The drawing under review shows one solid part. Ordinate dimensions are in mm from its lowest x, y, z. Coordinates: 2 decimals unless noted, no trailing zeros. Write each loop counter-clockwise with the first axis right and the second up, starting at its lowest first coordinate (ties: lowest second). Pieces come first, ordered by that corner, then holes.
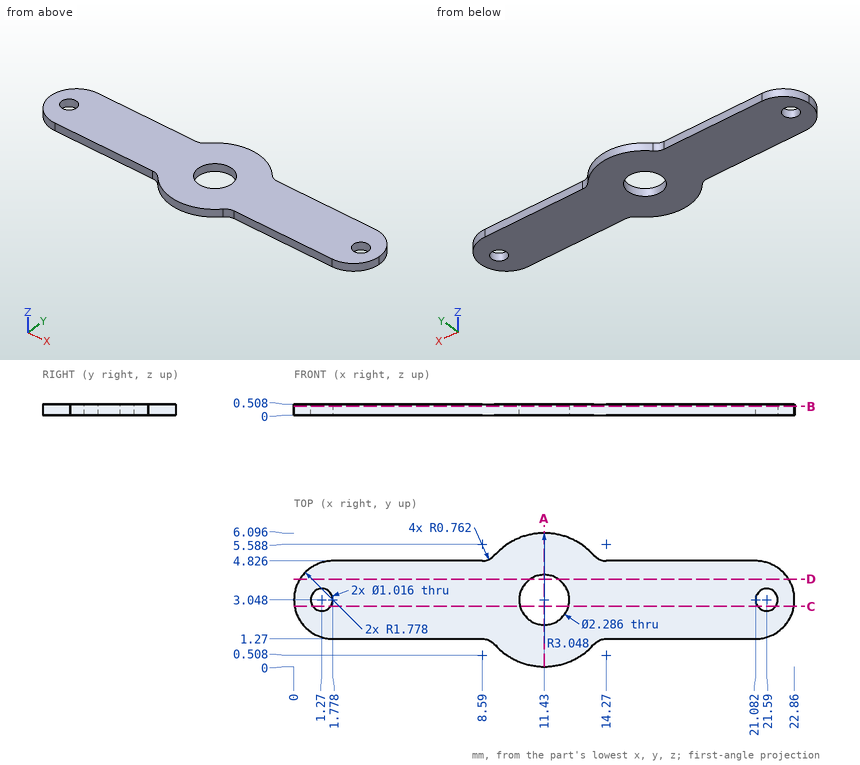
Q1. Add section C-C (y = 2.75). State the section outline as (x, z) points (1 decimal).
Ans:
outline: (0, 0) - (0.9, 0) - (0.9, 0.5) - (0, 0.5) - close; (1.7, 0) - (10.3, 0) - (10.3, 0.5) - (1.7, 0.5) - close; (12.5, 0) - (21.2, 0) - (21.2, 0.5) - (12.5, 0.5) - close; (22, 0) - (22.8, 0) - (22.8, 0.5) - (22, 0.5) - close
Q2. Add section D-D (y = 4). State the section outline as (x, z) points.
Ans:
outline: (0.28, 0) - (10.8, 0) - (10.8, 0.51) - (0.28, 0.51) - close; (12.06, 0) - (22.58, 0) - (22.58, 0.51) - (12.06, 0.51) - close
Q3. For probe 1 along Y at (x, z) = (11.43, 0.45) (3 decimals); probe 2 along Y at (x, z) = (21, 0.45); probe 3 along X at (y, z) = (3.5, 0.1), list the stretches that pass through material, from the lowest coordinate up.
Ans:
probe 1: y = 0 to 1.905, 4.191 to 6.096
probe 2: y = 1.27 to 4.83
probe 3: x = 0.06 to 1.04, 1.5 to 10.38, 12.48 to 21.36, 21.82 to 22.8
Q4. Add section B-B (z = 0.4). State the section outline as (x, y) points.
Ans:
outline: (1.78, 1.27) - (8.59, 1.27) arc R0.76 cw to (9.16, 1.02) arc R3.05 ccw to (13.7, 1.02) arc R0.76 cw to (14.27, 1.27) - (21.08, 1.27) arc R1.78 ccw to (21.08, 4.83) - (14.27, 4.83) arc R0.76 cw to (13.7, 5.08) arc R3.05 ccw to (9.16, 5.08) arc R0.76 cw to (8.59, 4.83) - (1.78, 4.83) arc R1.78 ccw to start; hole circle Ø1.02 at (1.27, 3.05); hole circle Ø2.29 at (11.43, 3.05); hole circle Ø1.02 at (21.59, 3.05)
Q5. Add section A-A (x = 11.43). State the section outline as (y, z) points (3 decimals).
Ans:
outline: (0, 0) - (1.905, 0) - (1.905, 0.508) - (0, 0.508) - close; (4.191, 0) - (6.096, 0) - (6.096, 0.508) - (4.191, 0.508) - close
